Autodesk Inventor part; units mm, degrees
ref_plane "YZ Plane" through (0, 0, 0) normal (1, 0, 0) x (0, 1, 0)
ref_plane "XZ Plane" through (0, 0, 0) normal (0, 1, 0) x (-1, 0, 0)
ref_plane "XY Plane" through (0, 0, 0) normal (0, 0, 1) x (1, 0, 0)
sketch "Эскиз1" plane through (-7.5, -11.4142, 0) normal (0, 0, 1) x (1, 0, 0)
  line L0 (0, 0) -> (0, 20)
  line L1 (0, 20) -> (2.8284, 22.8284)
  line L2 (0, 0) -> (15, 0)
  line L3 (15, 0) -> (15, 20)
  line L4 (15, 20) -> (12.1716, 22.8284)
  line L5 (12.1716, 22.8284) -> (2.8284, 22.8284)
  dimension "d5" = 20
  dimension "d4" = 4
  dimension "d3" = 135
  dimension "d2" = 15
  dimension "d1" = 4
  dimension "d0" = 135
revolve "Вращение1" add sketch "Эскиз1" angle 360 about axis through (-7.5, -11.4142, 0) along (1, 0, 0)
sketch "Эскиз2" plane through (7.5, -11.4142, 0) normal (1, 0, 0) x (0, 0, -1)
  circle A0 centre (0, 0) radius 20 construction
  point P0 (0, 11.4142)
hole "Отверстие1" at (7.5, -11.4142, 0) direction (-1, 0, 0) diameter 13 depth 6 tip angle 145 countersink diameter 16 countersink angle 60
properties part number "711131"
Design review of the part built by this model. Coordinates are the model's own, in mm. A direction names the side the tool comes from. Coordinates: 2 decimals unless noted, no trailing zeros. Write each loop counter-clockwise with the first axis right and the second up, starting at its lowest first coordinate (ties: lowest second). Pieces come first, ordered by that corner, then holes.
1) Machinability: for faces 5 (the conical face through (-7.32, -26.29, 13.64)), 6 (the cylindrical face through (3.18, -16.9, -3.49)), which of the approach directions +Z, -Z, +X, -X, +Y, -Y give a long, thin tool a straight path to every point of the face, cutting with its end or side? Answer none if there is none.
2) Add section A-A (x = -3.5). Write out the cut boundary in (y, z), plus the area to 3 significant figures.
3) Insertion check: pin 1 (4 mm diameter, centred on x = 3.5, y = -2.5, fed in from -Z); pin 2 (6 mm diameter, centred on x = 4, z = 12.5, fed in from -Y); pin 3 (1.5 mm diameter, centred on x = 2, z = 11, fed in from +Y). Each pin has a flat end and moves straight along its axis. Give the tip position at first contact, or say it passes through.
4) Add section B-B (x = 0.5). Write out the cut boundary in (y, z).
5) To check wall thickness, follow L1, parallel to Y at x = 3, z = -4; L2, parallel to X at y = 9, z = 7; L3, parallel to X at y = -14, z = 7.5. State the ranges of each line that lie inside material, in increasing order.
6) Mouldability with a two-part tool opening along Z and no side actions: class faces 1 (the cylindrical face through (-0.065, -16.363, 22.286)), 2 (the flat face through (-7.5, -12, 0)), 3 (the conical face through (5.1, -9.4, -6.3)), 4 (the conical face through (-0.42, -11.81, 0.09)) as +Z half, -Z half, draft (parallel to the pull), parting line (faces both ways), or undercut.
Check result:
1. face 5: -X
1. face 6: +X
2. outline: circle Ø45.66 at (-11.41, 0)
2. area: 1,640 mm2
3. pin 1: stops at z = -21.76
3. pin 2: stops at y = -32.17
3. pin 3: stops at y = 8.98
4. outline: circle Ø45.66 at (-11.41, 0); hole circle Ø6.66 at (-11.41, 0)
5. L1: y = -33.89 to -16.54, -6.29 to 11.06
5. L2: x = -5.92 to 5.92
5. L3: x = -7.5 to 7.38
6. face 1: parting line
6. face 2: draft
6. face 3: undercut
6. face 4: undercut
